Can you work these out from the model? Positions are in its coordinate system, mm. A direction names the side the tool comes from. Round coordinates to 2 decimals unless told otherwise and drop trailing zeros. Loops run counter-clockwise (first coordinate to the right, second up) from the corner with the lowest first, then second, coordinate; pieces in that order, holes last.
(1) Thinking about a two-plate mould opening in X: for faces 1 (the face through (6.751, 6.656, 26.447)), 2 (the face through (37.362, -33.075, 11.056)), 3 (the face through (25, -36, 7)), which applies, released by +X, released by -X, zero draft, split by the parting line, or undercut?
(2) Will these pins go through, and if not, where does the flat tip stop? pin 1 Ø2.5 at (y, z) = (-12.5, 9) entering from +X; pin 2 Ø8 at (x, z) = (20.5, 21) entering from -Y; pin 3 Ø8 at (x, y) = (19, -4.5) entering from +Z; pin 4 Ø9 at (y, z) = (-12, 9) entering from -X.
(3) I want a section at A-A on z = 11. Write out the boundary of the cut face in (x, y).
(4) I want a section at C-C on z = 28. Write out the boundary of the cut face in (x, y), plus the area to 4 significant figures.
(5) I want a section at B-B on x = 21. Write out the boundary of the cut face in (y, z).
(6) I want a section at D-D on y = -13. Write out the boundary of the cut face in (x, z), plus the area to 3 significant figures.
(7) Which directions (+Z, -Z, +X, -X, +Y, -Y) give clear straight access to the entire face, cutting with the end or side of a thin tool? Please do faces 4 (the face through (21, 7, 0)), 5 (the face through (0, 7, 21)), 6 (the face through (41.945, -10, 11)), 7 (the face through (25, -36, 15)), 8 (the face through (16, -45, 13)).
(8) If I drill on line 1 along Y through (x, z) = (21, 13); line 2 along X through (y, z) = (-20, 37.25); line 3 along X through (y, z) = (-46.5, 9), over which ranges is the centre line in solid material (lowest first)?
from build123d import *

# Parameters (mm, degrees)
F0_W     = 42
F0_H     = 10
F0_H_2   = 3.5
F1_DEPTH = 42
F2_R     = 1.75
F3_DEPTH = 25
F5_DEPTH = 8
F6_START = -27
F6_DEPTH = 8
F7_R     = 1.75
F8_DEPTH = 25


with BuildPart() as f1:
    # F0 (on Top) → F1 (new body)
    with BuildSketch(Plane.XY):
        with Locations((21, 5)):
            Rectangle(F0_W, F0_H)
        with Locations((21, 11.75)):
            Rectangle(F0_W, F0_H_2)
    extrude(amount=F1_DEPTH)

    # F2 (on face) → F3 (cut)
    with BuildSketch(Plane.XZ):
        with Locations((5.9434068862, 28)):
            Circle(F2_R)
        with Locations((5.9434068862, 4)):
            Circle(F2_R)
        with Locations((35.9434068862, 4)):
            Circle(F2_R)
        with Locations((35.9434068862, 28)):
            Circle(F2_R)
    extrude(amount=-F3_DEPTH, mode=Mode.SUBTRACT)

    # F4 (on face) → F5 (join)
    with BuildSketch(Plane.XY.offset(42)):
        with BuildLine():
            ThreePointArc((16, -35.1986841536), (11.6191684804, -7.0385186032), (37, -20))
            ThreePointArc((37, -20), (33.9614813968, -29.3808315196), (26, -35.1986841536))
            Line((26, -35.1986841536), (26, -40.33927218))
            ThreePointArc((26, -40.33927218), (37.4834789023, -32.9221095835), (41.9448321266, -20))
            ThreePointArc((41.9448321266, -20), (37.8665170629, -7.582005195), (27.219806493, 0))
            Line((27.219806493, 0), (14.780193507, 0))
            ThreePointArc((14.780193507, 0), (4.1334829371, -7.582005195), (0.0551678734, -20))
            ThreePointArc((0.0551678734, -20), (4.5165210977, -32.9221095835), (16, -40.33927218))
            Line((16, -40.33927218), (16, -35.1986841536))
        make_face()
        with BuildLine():
            Line((26, -40.33927218), (26, -35.1986841536))
            ThreePointArc((26, -35.1986841536), (24.0246055245, -35.7115168402), (22, -35.9687194227))
            Line((22, -35.9687194227), (22, -40.9209462695))
            ThreePointArc((22, -40.9209462695), (24.0140647283, -40.7268281853), (26, -40.33927218))
        make_face()
        with BuildLine():
            Line((26, -50.0102601945), (26, -40.33927218))
            ThreePointArc((26, -40.33927218), (24.0140647283, -40.7268281853), (22, -40.9209462695))
            Line((22, -40.9209462695), (22, -50.0102601945))
            Line((22, -50.0102601945), (26, -50.0102601945))
        make_face()
        with BuildLine():
            ThreePointArc((20, -40.9209462695), (17.9859352717, -40.7268281853), (16, -40.33927218))
            Line((16, -40.33927218), (16, -50.0102601945))
            Line((16, -50.0102601945), (20, -50.0102601945))
            Line((20, -50.0102601945), (20, -40.9209462695))
        make_face()
        with BuildLine():
            ThreePointArc((20, -35.9687194227), (17.9753944755, -35.7115168402), (16, -35.1986841536))
            Line((16, -35.1986841536), (16, -40.33927218))
            ThreePointArc((16, -40.33927218), (17.9859352717, -40.7268281853), (20, -40.9209462695))
            Line((20, -40.9209462695), (20, -35.9687194227))
        make_face()
        with BuildLine():
            ThreePointArc((22, -35.9687194227), (21, -36), (20, -35.9687194227))
            Line((20, -35.9687194227), (20, -40.9209462695))
            ThreePointArc((20, -40.9209462695), (21, -40.9448321266), (22, -40.9209462695))
            Line((22, -40.9209462695), (22, -35.9687194227))
        make_face()
        with BuildLine():
            ThreePointArc((22, -40.9209462695), (21, -40.9448321266), (20, -40.9209462695))
            Line((20, -40.9209462695), (20, -50.0102601945))
            Line((20, -50.0102601945), (22, -50.0102601945))
            Line((22, -50.0102601945), (22, -40.9209462695))
        make_face()
        with BuildLine():
            Line((0.0551678734, 0), (0.0551678734, -20))
            ThreePointArc((0.0551678734, -20), (4.1334829371, -7.582005195), (14.780193507, 0))
            Line((14.780193507, 0), (0.0551678734, 0))
        make_face()
        with BuildLine():
            ThreePointArc((27.219806493, 0), (37.8665170629, -7.582005195), (41.9448321266, -20))
            Line((41.9448321266, -20), (41.9448321266, 0))
            Line((41.9448321266, 0), (27.219806493, 0))
        make_face()
    extrude(amount=-F5_DEPTH)

    # F4 (on face) → F6 (join)
    with BuildSketch(Plane.XY.offset(42).offset(F6_START)):
        with BuildLine():
            ThreePointArc((16, -35.1986841536), (11.6191684804, -7.0385186032), (37, -20))
            ThreePointArc((37, -20), (33.9614813968, -29.3808315196), (26, -35.1986841536))
            Line((26, -35.1986841536), (26, -40.33927218))
            ThreePointArc((26, -40.33927218), (37.4834789023, -32.9221095835), (41.9448321266, -20))
            ThreePointArc((41.9448321266, -20), (37.8665170629, -7.582005195), (27.219806493, 0))
            Line((27.219806493, 0), (14.780193507, 0))
            ThreePointArc((14.780193507, 0), (4.1334829371, -7.582005195), (0.0551678734, -20))
            ThreePointArc((0.0551678734, -20), (4.5165210977, -32.9221095835), (16, -40.33927218))
            Line((16, -40.33927218), (16, -35.1986841536))
        make_face()
        with BuildLine():
            ThreePointArc((20, -35.9687194227), (17.9753944755, -35.7115168402), (16, -35.1986841536))
            Line((16, -35.1986841536), (16, -40.33927218))
            ThreePointArc((16, -40.33927218), (17.9859352717, -40.7268281853), (20, -40.9209462695))
            Line((20, -40.9209462695), (20, -35.9687194227))
        make_face()
        with BuildLine():
            ThreePointArc((20, -40.9209462695), (17.9859352717, -40.7268281853), (16, -40.33927218))
            Line((16, -40.33927218), (16, -50.0102601945))
            Line((16, -50.0102601945), (20, -50.0102601945))
            Line((20, -50.0102601945), (20, -40.9209462695))
        make_face()
        with BuildLine():
            Line((26, -50.0102601945), (26, -40.33927218))
            ThreePointArc((26, -40.33927218), (24.0140647283, -40.7268281853), (22, -40.9209462695))
            Line((22, -40.9209462695), (22, -50.0102601945))
            Line((22, -50.0102601945), (26, -50.0102601945))
        make_face()
        with BuildLine():
            Line((26, -40.33927218), (26, -35.1986841536))
            ThreePointArc((26, -35.1986841536), (24.0246055245, -35.7115168402), (22, -35.9687194227))
            Line((22, -35.9687194227), (22, -40.9209462695))
            ThreePointArc((22, -40.9209462695), (24.0140647283, -40.7268281853), (26, -40.33927218))
        make_face()
        with BuildLine():
            ThreePointArc((22, -40.9209462695), (21, -40.9448321266), (20, -40.9209462695))
            Line((20, -40.9209462695), (20, -50.0102601945))
            Line((20, -50.0102601945), (22, -50.0102601945))
            Line((22, -50.0102601945), (22, -40.9209462695))
        make_face()
        with BuildLine():
            ThreePointArc((22, -35.9687194227), (21, -36), (20, -35.9687194227))
            Line((20, -35.9687194227), (20, -40.9209462695))
            ThreePointArc((20, -40.9209462695), (21, -40.9448321266), (22, -40.9209462695))
            Line((22, -40.9209462695), (22, -35.9687194227))
        make_face()
        with BuildLine():
            Line((0.0551678734, 0), (0.0551678734, -20))
            ThreePointArc((0.0551678734, -20), (4.1334829371, -7.582005195), (14.780193507, 0))
            Line((14.780193507, 0), (0.0551678734, 0))
        make_face()
        with BuildLine():
            ThreePointArc((27.219806493, 0), (37.8665170629, -7.582005195), (41.9448321266, -20))
            Line((41.9448321266, -20), (41.9448321266, 0))
            Line((41.9448321266, 0), (27.219806493, 0))
        make_face()
    extrude(amount=-F6_DEPTH)

    # F7 (on face) → F8 (cut)
    with BuildSketch(Plane(origin=(16, 0, 0), x_dir=(0, -1, 0), z_dir=(-1, 0, 0))):
        with Locations((45.0102601945, 38)):
            Circle(F7_R)
        with Locations((45.0102601945, 11)):
            Circle(F7_R)
    extrude(amount=-F8_DEPTH, mode=Mode.SUBTRACT)


solid = f1.part
Filled sheet:
1. face 1: undercut
1. face 2: released by +X
1. face 3: zero draft
2. pin 1: stops at x = 41.94
2. pin 2: stops at y = 0
2. pin 3: stops at z = 42
2. pin 4: stops at x = 0.06
3. outline: (0, 0) - (0.06, 0) - (0.06, -20) arc R20.94 ccw to (16, -40.34) - (16, -43.26) - (26, -43.26) - (26, -40.34) arc R20.94 ccw to (41.94, -20) - (41.94, 0) - (42, 0) - (42, 13.5) - (0, 13.5) - close; (16, -50.01) - (26, -50.01) - (26, -46.76) - (16, -46.76) - close; hole circle Ø32 at (21, -20)
4. outline: (0, 0) - (4.19, 0) - (4.19, 13.5) - (0, 13.5) - close; (7.69, 0) - (34.19, 0) - (34.19, 13.5) - (7.69, 13.5) - close; (37.69, 0) - (42, 0) - (42, 13.5) - (37.69, 13.5) - close
4. area: 472.5 mm2
5. outline: (-50.01, 7) - (-36, 7) - (-36, 15) - (-50.01, 15) - close; (-50.01, 34) - (-36, 34) - (-36, 42) - (-50.01, 42) - close; (-4, 7) - (0, 7) - (0, 0) - (13.5, 0) - (13.5, 42) - (-4, 42) - (-4, 34) - (0, 34) - (0, 15) - (-4, 15) - close; hole circle Ø3.5 at (-45.01, 11); hole circle Ø3.5 at (-45.01, 38)
6. outline: (0.06, 7) - (6.61, 7) - (6.61, 15) - (0.06, 15) - close; (0.06, 34) - (6.61, 34) - (6.61, 42) - (0.06, 42) - close; (35.39, 7) - (41.94, 7) - (41.94, 15) - (35.39, 15) - close; (35.39, 34) - (41.94, 34) - (41.94, 42) - (35.39, 42) - close
6. area: 210 mm2
7. face 4: -Z, +X, -X, +Y, -Y
7. face 5: +Z, -Z, -X, +Y, -Y
7. face 6: +Z, -Z, +X, -Y
7. face 7: +X, -X, -Y
7. face 8: +Z, -Z, -X, -Y
8. line 1: y = -50.01 to -36, -4 to 13.5
8. line 2: x = 0.06 to 5, 37 to 41.94
8. line 3: x = 16 to 26
